Work out the finished part from the listing and answer in its coordinate system (mm). A direction names the side the tool comes from. Give positions to 0.01 mm unless a question says otherwise; leave off trailing zeros. Order: outer loops, then holes, each group sorted by start corner. A loop starts at its lowest first (then second) coordinate and runs counter-clockwise, first axis right, second up. Notation, with made-up numbers: (46, 58.5) - (62, 58.5) arc R28 ccw to (62, 76.5) - close; hole circle Ø1 at (32, -6). An arc over 180 degrees is marked (long way). Put each result on its own line as item: value.
```python
from build123d import *

# Parameters (mm, degrees)
EXTRUDE_1_DEPTH     = 30
SKETCH_2_W          = 7
SKETCH_2_H          = 35
EXTRUDE_2_DEPTH     = 4
CUT_EXTRUDE_1_DEPTH = 6
SKETCH_4_W          = 17.5
SKETCH_4_H          = 4
EXTRUDE_3_DEPTH     = 23


with BuildPart() as part:
    # Эскиз1 → Бобышка-Вытянуть1 (new body)
    with BuildSketch(Plane.XY):
        Polygon((4, 0), (-4, 0), (-4, -1.5), (-8.75, -1.5), (-8.75, -3), (-4, -6.5), (4, -6.5), (8.75, -3), (8.75, -1.5), (4, -1.5), align=None)
    extrude(amount=EXTRUDE_1_DEPTH)

    # Эскиз2 → Бобышка-Вытянуть2 (add, symmetric)
    with BuildSketch(Plane(origin=(0, 0, 0), x_dir=(0, 0, -1), z_dir=(1, 0, 0))):
        with Locations((-26.5, 11)):
            Rectangle(SKETCH_2_W, SKETCH_2_H)
    extrude(amount=EXTRUDE_2_DEPTH, both=True)

    # Эскиз3 → Вырез-Вытянуть1 (cut, through all)
    with BuildSketch(Plane(origin=(0, -1.5, 0), x_dir=(1, 0, 0), z_dir=(0, 1, 0))):
        Polygon((-4, 0), (-8.75, -2.742413779), (-8.75, 0), align=None)
        Polygon((-4, -28), (-8.75, -23.25), (-8.75, -30), (-4, -30), align=None)
        Polygon((4, -30), (4, -28), (8.75, -23.25), (8.75, -30), align=None)
        Polygon((8.75, 0), (4, 0), (8.75, -2.742413779), align=None)
    extrude(amount=-CUT_EXTRUDE_1_DEPTH, mode=Mode.SUBTRACT)

    # Эскиз4 → Бобышка-Вытянуть3 (add)
    with BuildSketch(Plane(origin=(0, 28.5, 0), x_dir=(1, 0, 0), z_dir=(0, 1, 0))):
        with Locations((0, -26.5)):
            Rectangle(SKETCH_4_W, SKETCH_4_H)
    extrude(amount=-EXTRUDE_3_DEPTH)

    # Эскиз6 → Отверстие обработанное метчиком M61 (revolve, cut)
    with BuildSketch(Plane(origin=(0, -6.5, 10), x_dir=(0, 0, -1), z_dir=(1, 0, 0))):
        Polygon((0, 0), (0, 6.5), (3.1, 6.5), (2.5, 5.9), (2.5, 0.6), (3.1, 0), align=None)
    revolve(axis=Axis((0, -12.85, 10), (0, 1, 0)), mode=Mode.SUBTRACT)

    # Эскиз8 → Отверстие обработанное метчиком M62 (revolve, cut)
    with BuildSketch(Plane(origin=(0, 17.5, 30), x_dir=(0, -1, 0), z_dir=(1, 0, 0))):
        Polygon((0, 0), (0, 7), (3.1, 7), (2.5, 6.4), (2.5, 0.6), (3.1, 0), align=None)
    revolve(axis=Axis((0, 17.5, 36.35), (0, 0, -1)), mode=Mode.SUBTRACT)


solid = part.part
```
(1) Section D-D, the plane y = -1 is taken. Write down the section's boundary in (x, z), then the cut area to 3 significant figures.
Geometry check:
outline: (-4, 0) - (4, 0) - (4, 30) - (-4, 30) - close; hole circle Ø5 at (0, 10)
area: 220 mm²
(2) Section C-C, the plane y = 17.5 is taken. Write down the section's boundary in (x, z), then the cut area to 3 significant figures.
Geometry check:
outline: (-8.75, 24.5) - (-4, 24.5) - (-4, 23) - (-3.1, 23) - (-2.5, 23.6) - (-2.5, 29.4) - (-3.1, 30) - (-4, 30) - (-4, 28.5) - (-8.75, 28.5) - close; (2.5, 23.6) - (3.1, 23) - (4, 23) - (4, 24.5) - (8.75, 24.5) - (8.75, 28.5) - (4, 28.5) - (4, 30) - (3.1, 30) - (2.5, 29.4) - close
area: 58.3 mm²
(3) A tool of negligible diameter and unlimited length cuts with its end or side. For faces 4 (the face through (6, 17, 28.5)), 5 (the face through (-6, 17, 24.5)), 6 (the face through (-6, -3, 26)), 7 (the face through (0, 0, 14)), 8 (the face through (6, -3, 26)), from which of +Z, -Z, +X, -X, +Y, -Y can it reach the whole face along a straight path? Write none if from no direction.
Geometry check:
face 4: +Z, +X, +Y, -Y
face 5: -Z, -X, +Y
face 6: +Z, -X, -Y
face 7: -Z, +X, -X, +Y
face 8: +Z, +X, -Y
(4) Section A-A, the plane z = 10 is taken. Write down the section's boundary in (x, y).
Geometry check:
outline: (-8.75, -3) - (-4, -6.5) - (-3.1, -6.5) - (-2.5, -5.9) - (-2.5, -0.6) - (-3.1, 0) - (-4, 0) - (-4, -1.5) - (-8.75, -1.5) - close; (2.5, -5.9) - (3.1, -6.5) - (4, -6.5) - (8.75, -3) - (8.75, -1.5) - (4, -1.5) - (4, 0) - (3.1, 0) - (2.5, -0.6) - close
(5) Given pin 1 (5 mm diameter, centred on x = -5.5, y = 15, fed in from +Z); pin 2 (1.2 mm diameter, centred on x = 7.5, z = 27.5, fed in from -Y); pin 3 (2.5 mm diameter, centred on x = -1, z = 13, fed in from +Y); pin 4 (5 mm diameter, centred on x = -7, y = 19.5, fed in from -Z), each flat-ended and moving along its own axis, determine where each tip first touches the part or whether it passes through.
Geometry check:
pin 1: stops at z = 30
pin 2: stops at y = 5.5
pin 3: stops at y = 0
pin 4: stops at z = 24.5
(6) Section B-B, the plane x = 0 is taken. Write down the section's boundary in (y, z).
Geometry check:
outline: (-6.5, 0) - (0, 0) - (0, 6.9) - (-0.6, 7.5) - (-5.9, 7.5) - (-6.5, 6.9) - close; (-6.5, 13.1) - (-5.9, 12.5) - (-0.6, 12.5) - (0, 13.1) - (0, 23) - (14.4, 23) - (15, 23.6) - (15, 29.4) - (14.4, 30) - (-6.5, 30) - close; (20, 23.6) - (20.6, 23) - (28.5, 23) - (28.5, 30) - (20.6, 30) - (20, 29.4) - close
(7) Determine the mould class of faces 1 (the face through (8.75, -2, 13)), 2 (the face through (0, 28.5, 26)), 3 (the face through (-4, 7, 24)) for opening direction Y: pulls with the +Y half, pulls with the -Y half, needs draft (parallel to the pull), parting line crosses it, or undercut.
Geometry check:
face 1: needs draft
face 2: pulls with the +Y half
face 3: undercut
(8) Straight lines are drawn through the part: line 1 (Y direction, x = 0, z = 25.75); line 2 (Z direction, x = 0, y = -2.35); line 3 (X direction, y = 17.5, z = 25.15). For each, find the intervals that lie inside material, in ascending order.
Geometry check:
line 1: y = -6.5 to 15, 20 to 28.5
line 2: z = 0 to 7.5, 12.5 to 30
line 3: x = -8.75 to -2.5, 2.5 to 8.75
